Design review of the part built by this model. Coordinates are the model's own, in mm. A direction names the side the tool comes from. Give positions to 0.01 mm unless a question says otherwise; leave off trailing zeros. Loops run counter-clockwise (first coordinate to the right, second up) from the corner with the lowest first, then second, coordinate; pieces in that order, holes last.
Autodesk Inventor part; units mm, degrees
ref_plane "YZ Plane" through (0, 0, 0) normal (1, 0, 0) x (0, 1, 0)
ref_plane "XZ Plane" through (0, 0, 0) normal (0, 1, 0) x (-1, 0, 0)
ref_plane "XY Plane" through (0, 0, 0) normal (0, 0, 1) x (1, 0, 0)
sketch "Sketch1" plane through (0, 0, 0) normal (0, 1, 0) x (-1, 0, 0)
  circle A0 centre (0, 0) radius 1.4
  circle A1 centre (0, 0) radius 5
  circle A2 centre (0, 0) radius 1.115
  dimension "d0" = 2.8
  dimension "d1" = 10
extrude "Extrusion1" add sketch "Sketch1" along normal blind 16 contours A0 | A1 | A2
extrude "Extrusion2" cut sketch "Sketch1" along normal blind 8 contours A0 | A2
sketch "Sketch2" plane through (0, 16, 0) normal (0, 1, 0) x (1, 0, 0)
  circle A0 centre (0, 0) radius 3 construction
  circle A1 centre (0, 0) radius 3.19
  line L0 (-2.8414, 1.45) -> (2.8414, 1.45) construction
  line L1 (-2.7421, 1.63) -> (2.7421, 1.63)
  point P0 (0, -3)
  dimension "d6" = 6
  dimension "d7" = 6.38
  dimension "d8" = 4.45
  dimension "d9" = 0.18
extrude "Extrusion3" cut sketch "Sketch2" against normal blind 6 contours A1 L1 picked at (0.1058, 0.0286)
properties part number "Motor Rotary Encoder Coupler"
Q1. Wall thickness on line 1 (Z direction, x = 0, y = 14.6); line 2 (Z direction, x = 0, y = 4); line 3 (Y direction, x = -2, z = -0.75): over which ranges is each line inside the solid? List them lowest first.
Results:
line 1: z = -5 to -1.63, 3.19 to 5
line 2: z = -5 to -1.4, 1.4 to 5
line 3: y = 0 to 10
Q2. Insertion check: pin 1 (1 mm diameter, centred on x = -2, y = 13.5, fed in from +Z); pin 2 (1.4 mm diameter, centred on x = 0.5, z = 0, fed in from -Y); pin 3 (2.5 mm diameter, centred on x = 0, z = 0, fed in from +Y). Each pin has a flat end and moves straight along its axis. Give the tip position at first contact, or say it passes through.
Results:
pin 1: stops at z = 4.77
pin 2: stops at y = 8
pin 3: stops at y = 10
Q3. Tool access review of faces 4 (the face through (-1, 0, 1.2)), 5 (the face through (1.4, 3.94, -0.06)), 6 (the face through (0, 10, 1)): name each direction out of +Z, -Z, +X, -X, +Y, -Y from which nothing blocks a thin tool from reaching the whole face with its end or side.
Results:
face 4: +Z, -Z, +X, -X, -Y
face 5: -Y
face 6: +Y
Q4. Take a section at C-C (y = 1.75). Give the boundary of the cut face in (x, z).
Results:
outline: circle Ø10 at (0, 0); hole circle Ø2.8 at (0, 0)
Q5. Draft analysis for pull direction X (two halves, no side actions). For faces 1 (the face through (-0.09, 13.04, 3.19)), 2 (the face through (0, 16, -2)), 3 (the face through (1.08, 7.89, 4.88)), state which applies: pulls with the +X half, pulls with the -X half, needs draft (parallel to the pull), parting line crosses it, or undercut.
Results:
face 1: undercut
face 2: needs draft
face 3: parting line crosses it
Q6. Take a section at B-B (x = 0). Give the boundary of the cut face in (y, z).
Results:
outline: (0, -5) - (16, -5) - (16, -1.63) - (10, -1.63) - (10, 3.19) - (16, 3.19) - (16, 5) - (0, 5) - (0, 1.4) - (8, 1.4) - (8, -1.4) - (0, -1.4) - close
Q7. Take a section at D-D (y = 9). Give the boundary of the cut face in (x, z), plus the area to 3 significant figures.
Results:
outline: circle Ø10 at (0, 0)
area: 78.5 mm2
Q8. Take a section at A-A (z = 0). Give the boundary of the cut face in (x, y).
Results:
outline: (-5, 0) - (-1.4, 0) - (-1.4, 8) - (1.4, 8) - (1.4, 0) - (5, 0) - (5, 16) - (3.19, 16) - (3.19, 10) - (-3.19, 10) - (-3.19, 16) - (-5, 16) - close
